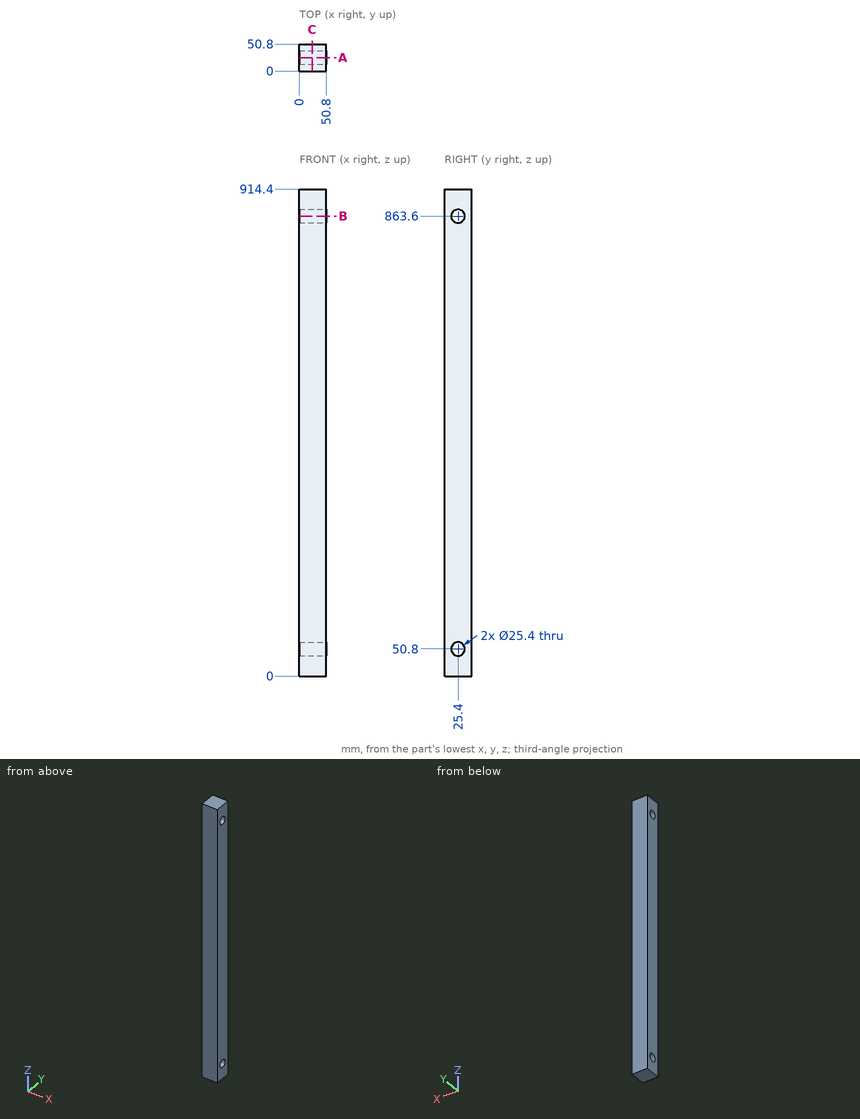
Check sheet for the drawn part. Datum: minimum x, y, z corner. Units: mm. Give positions to 0.01 mm unless a question says otherwise; leave off trailing zeros. Order: outer loops, then holes, each group sorted by start corner. A loop starts at its lowest first (then second) coordinate and runs counter-clockwise, first axis right, second up. Notation, with made-up numbers: (44.5, 88.5) -> (74.5, 88.5) arc R17 cw to (74.5, 98.5) -> close; hole circle Ø4 at (48.5, 4). An arc over 180 degrees is marked (long way). Use a Markdown table: item, result.
1) Section check A-A, the plane y = 25.4. Record the boundary of the cut face in (x, z).
Results:
| item | result |
|---|---|
| outline | (0, 0) -> (50.8, 0) -> (50.8, 38.1) -> (0, 38.1) -> close; (0, 63.5) -> (50.8, 63.5) -> (50.8, 850.9) -> (0, 850.9) -> close; (0, 876.3) -> (50.8, 876.3) -> (50.8, 914.4) -> (0, 914.4) -> close |
2) Section check C-C, the plane x = 24. Record the boundary of the cut face in (y, z), then the cut area to 3 significant figures.
Results:
| item | result |
|---|---|
| outline | (0, 0) -> (50.8, 0) -> (50.8, 914.4) -> (0, 914.4) -> close; hole circle Ø25.4 at (25.4, 50.8); hole circle Ø25.4 at (25.4, 863.6) |
| area | 45,400 mm² |
3) Material ranges on probe 1 along Z at (x, y) = (21, 25); probe 2 along Z at (x, y) = (39, 27.5); probe 3 along Y at (x, z) = (40, 863), recorded low to high.
Results:
| item | result |
|---|---|
| probe 1 | 0 to 38.11, 63.49 to 850.91, 876.29 to 914.4 |
| probe 2 | 0 to 38.27, 63.33 to 851.07, 876.13 to 914.4 |
| probe 3 | 0 to 12.71, 38.09 to 50.8 |
4) Section check B-B, the plane z = 863.6. Record the boundary of the cut face in (x, y).
Results:
| item | result |
|---|---|
| outline | (0, 0) -> (50.8, 0) -> (50.8, 12.7) -> (0, 12.7) -> close; (0, 38.1) -> (50.8, 38.1) -> (50.8, 50.8) -> (0, 50.8) -> close |
